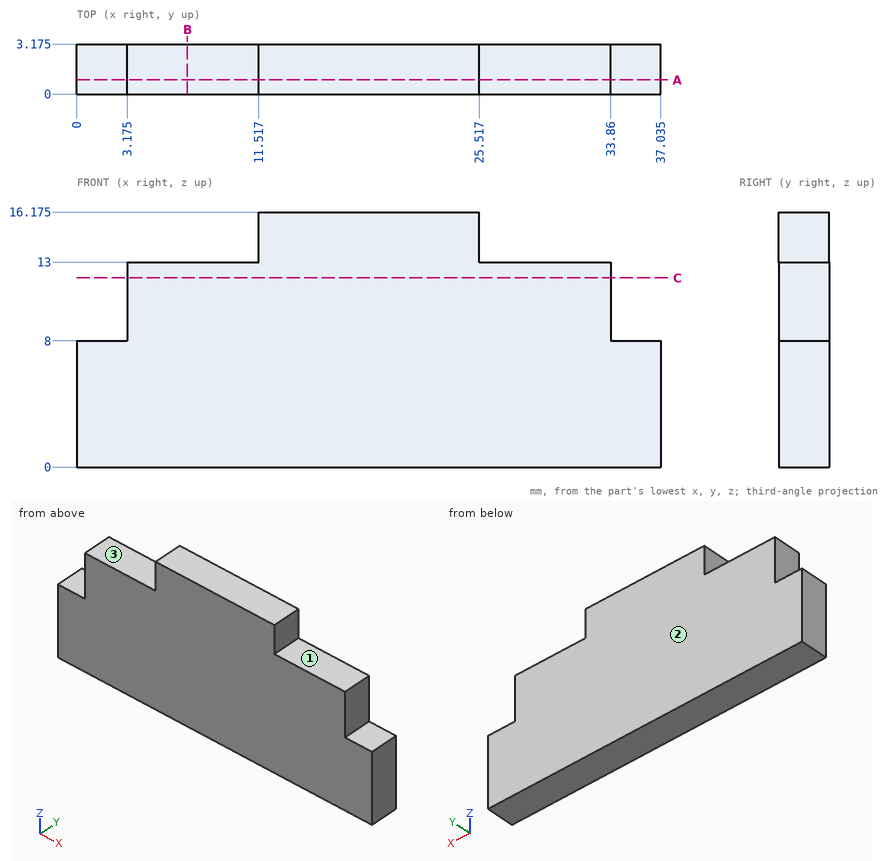
Source: three-view drawing plus pictorial views. Frame: mm from the lowest corner of the part. A direction names the side the tool comes from. Give positions to 0.01 mm unless a question says otherwise; leave off trailing zeros. Loops run counter-clockwise (first coordinate to the right, second up) from the corner with the lowest first, then second, coordinate; pieces in that order, holes last. Notation, with made-up numbers: (28, 22) -> (65, 22) arc R23 ccw to (65, 44) -> close; hole circle Ø3 at (69, 82). An arc over 180 degrees is marked (long way). Use a Markdown table: item, result. Add a question column.
(1) Section query B-B (x = 7). Output: boundary loops of the cut face in (y, z) (1 decimal).
(2) Section query A-A (y = 0.9). Output: boundary loops of the cut face in (x, z) (1 decimal), then the cut area to 3 significant figures.
(3) Section query C-C (z = 12). Output: boundary loops of the cut face in (x, y) (1 decimal).
(4) Ray query, line 1 (Z direction, x = 2, y = 1.6); line 2 (X direction, y = 1.4, z = 14.75); line 3 (Z direction, x = 31.5, y = 2.4). Return the intervals inside material, ascending.
(5) Access query for the marked faces 1, 2 and 3. Directions: +Z, -Z, +X, -X, +Y, -Y. A direction counts if a zero-diameter tool reaches every point of the face in a straight line with its end or side. Return the directions, or none.
(6) First-contact query: pin 1 Ø1.6 at (y, z) = (2, 11.5) entering from +X; pin 2 Ø1.6 at (x, y) = (30.5, 2) entering from +Z; pin 3 Ø1.6 at (y, z) = (1.5, 11) entering from -X (3 decimals). Flat tips, straight axial feed; report the tip coordinate or a pass-through.
Checked values:
| question | item | result |
|---|---|---|
| 1 | outline | (0, 0) -> (3.2, 0) -> (3.2, 13) -> (0, 13) -> close |
| 2 | outline | (0, 0) -> (37, 0) -> (37, 8) -> (33.9, 8) -> (33.9, 13) -> (25.5, 13) -> (25.5, 16.2) -> (11.5, 16.2) -> (11.5, 13) -> (3.2, 13) -> (3.2, 8) -> (0, 8) -> close |
| 2 | area | 494 mm^2 |
| 3 | outline | (3.2, 0) -> (33.9, 0) -> (33.9, 3.2) -> (3.2, 3.2) -> close |
| 4 | line 1 | 0 to 8 |
| 4 | line 2 | 11.52 to 25.52 |
| 4 | line 3 | 0 to 13 |
| 5 | face 1 | +Z, +X, +Y, -Y |
| 5 | face 2 | +Z, -Z, +X, -X, +Y |
| 5 | face 3 | +Z, -X, +Y, -Y |
| 6 | pin 1 | x = 33.86 |
| 6 | pin 2 | z = 13 |
| 6 | pin 3 | x = 3.175 |
